Check sheet for the modelled part. Datum: model origin and axes. Units: mm. A direction names the side the tool comes from. Round coordinates to 2 decimals unless told otherwise and drop trailing zeros. Order: outer loops, then holes, each group sorted by start corner. A loop starts at its lowest first (then second) coordinate and runs counter-clockwise, first axis right, second up.
(1) Thickness scan on probe 1 along Z at (x, y) = (-5, -32.5); probe 2 along Z at (x, y) = (32, -20); probe 3 along X at (y, z) = (-10, 11.5). Record the ranges inside material, lowest first.
(2) Sectioned sample at A-A, the plane x = 0. Enter the section's corners in (y, z).
(3) Sectioned sample at D-D, the plane z = 32. Enter the section's corners in (x, y), and give its area (3 significant figures).
(4) Depth check by flat-ended pin: pin 1 (2 mm diameter, centred on y = 27.5, z = 41.5, fed in from -X); pin 2 (6 mm diameter, centred on y = -21.5, z = 26, fed in from -X); pin 3 (3 mm diameter, centred on x = 28.5, z = 41.5, fed in from -Y); pin 4 (1.5 mm diameter, centred on y = -24, z = 33, fed in from -X) (1 decimal). Enter the tip coordinate at first touch or a pass-through.
(5) Mould release check, pull along Z, two halves, no side actions. Record for faces 3 (the flat face through (0, 0, 60)), 4 (the cylindrical face through (-8.67, -39.05, 47.78)), 5 (the flat face through (0, 8, 35.362)), 6 (the flat face through (0, 0, 0)): released by +Z, released by -Z, zero draft, split by the parting line, or undercut.
(6) Sectioned sample at C-C, the plane z = 41.5. Enter the section's corners in (x, y).
(7) Tool access check on faces 1 (the cylindrical face through (-7.493, 0.33, 30.075)), 2 (the cylindrical face through (-8.67, -39.05, 12.22)). Record the directions out of +Z, -Z, +X, -X, +Y, -Y that give a thin tool (end or side, any length) a straight path to the whole face; none if there is none.
```python
from build123d import *

# Parameters (mm, degrees)
F0_R     = 40
F1_DEPTH = 24.638
F2_R     = 5.08
F3_R     = 7.5
F4_DEPTH = 30


with BuildPart() as f1:
    # F0 (on Top) → F1 (new body)
    with BuildSketch(Plane.XY):
        Circle(F0_R)
    extrude(amount=F1_DEPTH)

    # F2
    f2_edges = [f1.edges().sort_by_distance(p)[0] for p in [
        (-40, 0, 24.638),
        (-40, 0, 0),
    ]]
    fillet(f2_edges, radius=F2_R)

    # F3 (on Top) → F4 (join)
    with BuildSketch(Plane.XY):
        Circle(F3_R)
    extrude(amount=F4_DEPTH)

    # F5: F1 across face


with BuildPart() as f1_1:
    add(f1.part)
    add(f1.part.mirror(Plane.XY.offset(30)))


solid = f1_1.part
```
Derived:
1. probe 1: z = 0 to 24.64, 35.36 to 60
1. probe 2: z = 0.85 to 23.79, 36.21 to 59.15
1. probe 3: x = -38.73 to 38.73
2. outline: (-40, 5.08) arc R5.08 ccw to (-34.92, 0) - (34.92, 0) arc R5.08 ccw to (40, 5.08) - (40, 19.56) arc R5.08 ccw to (34.92, 24.64) - (7.5, 24.64) - (7.5, 35.36) - (34.92, 35.36) arc R5.08 ccw to (40, 40.44) - (40, 54.92) arc R5.08 ccw to (34.92, 60) - (-34.92, 60) arc R5.08 ccw to (-40, 54.92) - (-40, 40.44) arc R5.08 ccw to (-34.92, 35.36) - (-7.5, 35.36) - (-7.5, 24.64) - (-34.92, 24.64) arc R5.08 ccw to (-40, 19.56) - close
3. outline: circle Ø15 at (0, 0)
3. area: 177 mm2
4. pin 1: stops at x = -29.96
4. pin 2: stops at x = -32.61
4. pin 3: stops at y = -29.51
4. pin 4: passes through
5. face 3: released by +Z
5. face 4: zero draft
5. face 5: undercut
5. face 6: released by -Z
6. outline: circle Ø80 at (0, 0)
7. face 1: none
7. face 2: +Z, -Z
